Part print with two shaded views. Sizes in mm from the minimum x, y, z corner. A direction names the side the tool comes from. Round coordinates to 2 decimals unless told otherwise and drop trailing zeros. Loops run counter-clockwise (first coordinate to the right, second up) from the corner with the lowest first, then second, coordinate; pieces in that order, holes last. Notation, with made-up numbers: (43, 1) -> (88, 1) arc R12 ccw to (88, 12) -> close; hole circle Ø5 at (79.25, 17). An arc over 180 degrees is marked (long way). Use a Markdown table: item, result. Add a question column.
Item 1: Which spindle directions (+Z, -Z, +X, -X, +Y, -Y) get a long thin tool onto all of the face, cutting with end or side? Do the marked faces 1 and 2. Say none if no direction does.
Item 2: Cut at A-A, the plane z = 3. List the corners of the cut face in (x, y), plus the area to 3 significant figures.
Item 3: Cut at D-D, the plane x = 1.25. List the corners of the cut face in (y, z).
Item 4: Two-plate mould, pull along Y, no slides. Class the marked faces 3, 4 and 5: pulls with the +Y half, pulls with the -Y half, needs draft (parallel to the pull), parting line crosses it, or undercut.
Item 5: Cut at B-B, the plane x = 6. List the corners of the cut face in (y, z), plus the area to 3 significant figures.
Item 6: Cut at C-C, the plane y = 3. List the corners of the cut face in (x, z), plus the area to 3 significant figures.
Item 7: Probe line 1 (Y direction, x = 3.25, z = 3); line 2 (Y direction, x = 6.25, z = 4.75); line 3 (Z direction, x = 1, y = 2). List the from-to ranges inside material, lowest first. Write a range as [from, to].
Item 8: Flat gauge pins, fed straight in: pin 1 (0.5 mm diameter, centred on x = 6, z = 4.5, fed in from +Y); pin 2 (0.5 mm diameter, centred on y = 3, z = 5, fed in from +X); pin 3 (1.5 mm diameter, centred on x = 5.5, z = 1.5, fed in from -Y); pin 4 (1.5 mm diameter, centred on y = 1.5, z = 5, fed in from -X). Where does each tip first touch, or does it go through?
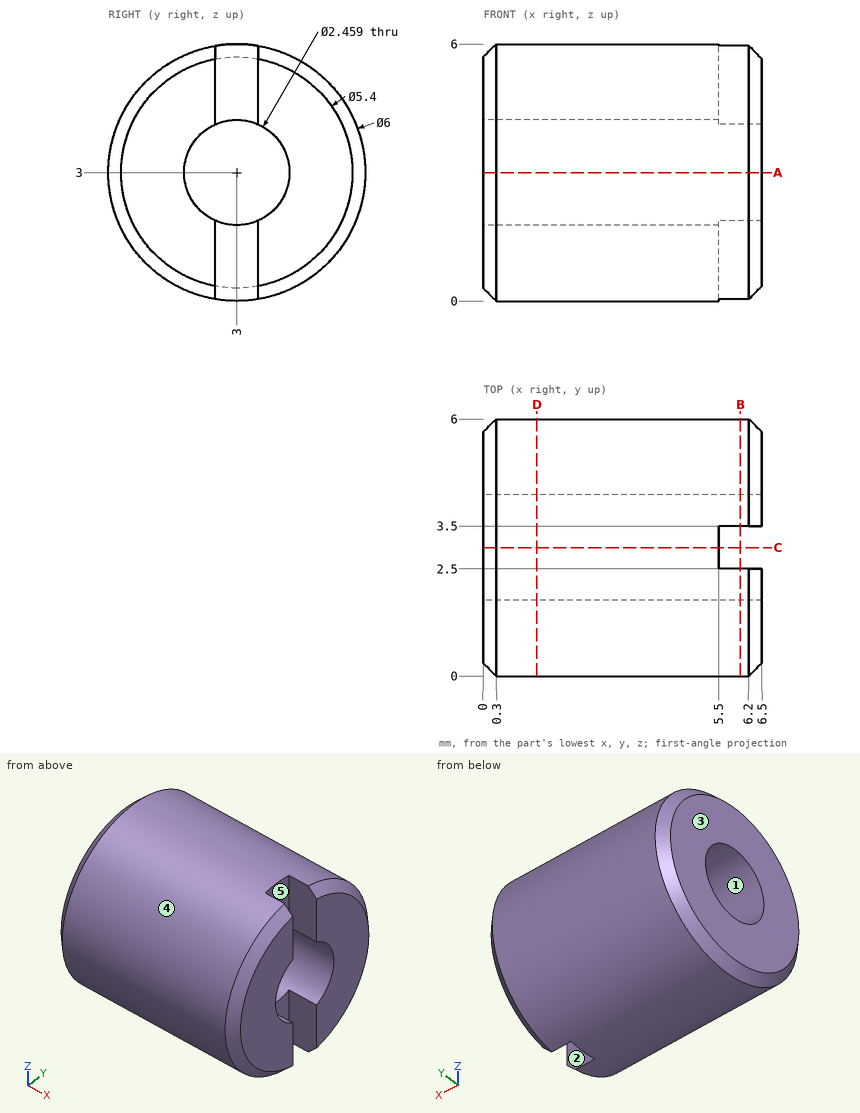
A:
| question | item | result |
|---|---|---|
| 1 | face 1 | +X, -X |
| 1 | face 2 | +Z, -Z, +X |
| 2 | outline | (0, 0.3) -> (0.3, 0) -> (6.2, 0) -> (6.5, 0.3) -> (6.5, 1.77) -> (0, 1.77) -> close; (0, 4.23) -> (6.5, 4.23) -> (6.5, 5.7) -> (6.2, 6) -> (0.3, 6) -> (0, 5.7) -> close |
| 2 | area | 22.8 mm^2 |
| 3 | outline | circle Ø6 at (3, 3); hole circle Ø2.46 at (3, 3) |
| 4 | face 3 | needs draft |
| 4 | face 4 | parting line crosses it |
| 4 | face 5 | undercut |
| 5 | outline | (2.5, 0.04) -> (2.5, 1.88) arc R1.23 cw to (2.5, 4.12) -> (2.5, 5.96) arc R3 ccw to start; (3.5, 0.04) arc R3 ccw to (3.5, 5.96) -> (3.5, 4.12) arc R1.23 cw to (3.5, 1.88) -> close |
| 5 | area | 19.9 mm^2 |
| 6 | outline | (0, 0.3) -> (0.3, 0) -> (5.5, 0) -> (5.5, 1.77) -> (0, 1.77) -> close; (0, 4.23) -> (5.5, 4.23) -> (5.5, 6) -> (0.3, 6) -> (0, 5.7) -> close |
| 6 | area | 19.4 mm^2 |
| 7 | line 1 | y = [0, 1.77], [4.23, 6] |
| 7 | line 2 | y = [0.63, 2.5], [3.5, 5.37] |
| 7 | line 3 | z = [0.17, 2.28], [3.72, 5.83] |
| 8 | pin 1 | stops at y = 5.73 |
| 8 | pin 2 | stops at x = 5.5 |
| 8 | pin 3 | stops at y = 0.1 |
| 8 | pin 4 | stops at x = 0 |
